Check sheet for the drawn part. Datum: minimum x, y, z corner. Units: mm. A direction names the side the tool comes from. Give positions to 0.01 mm unless a question says otherwise; leave off trailing zeros. Order: outer loops, then holes, each group sorted by start corner. A loop starts at its lowest first (then second) coordinate and runs counter-clockwise, first axis right, second up.
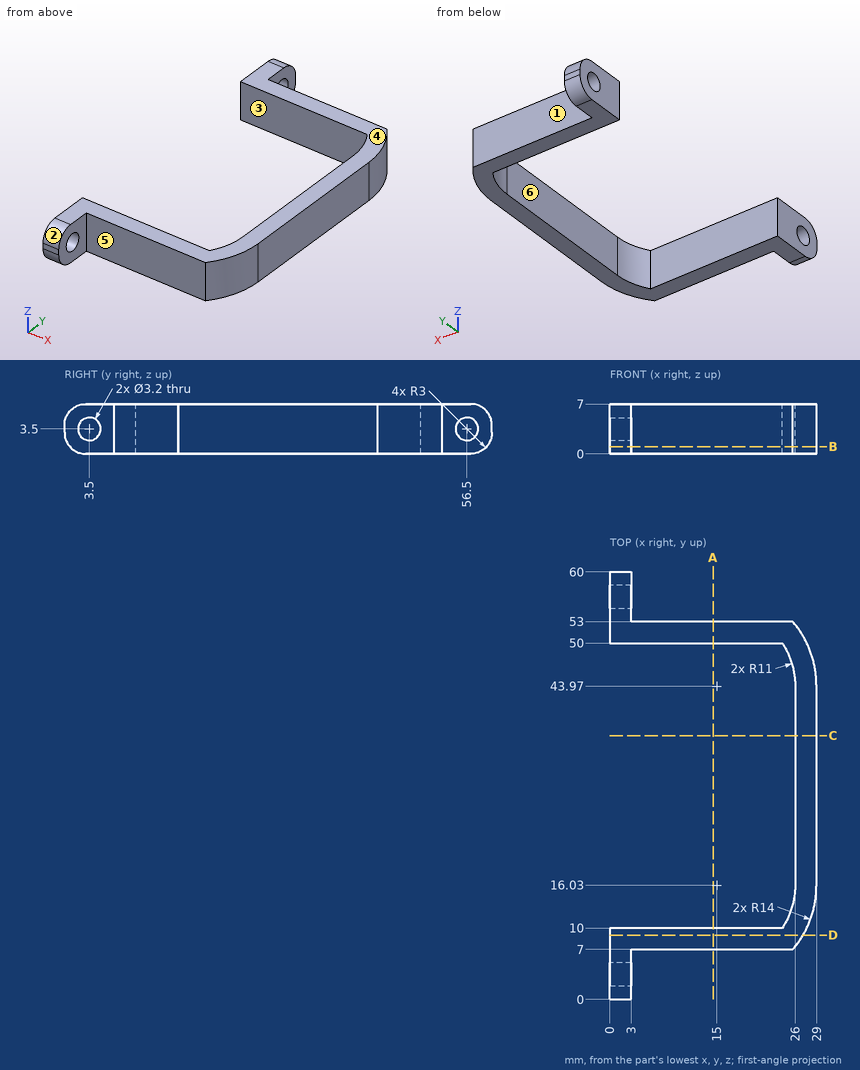
(1) Section check B-B, the plane z = 1. Enter the section's corners in (x, y).
Solved:
outline: (0, 0.76) - (3, 0.76) - (3, 7) - (25.7, 7) arc R14 ccw to (29, 16) - (29, 44) arc R14 ccw to (25.7, 53) - (3, 53) - (3, 59.24) - (0, 59.24) - (0, 50) - (24.2, 50) arc R11 cw to (26, 43.94) - (26, 16.06) arc R11 cw to (24.2, 10) - (0, 10) - close
(2) Section check A-A, the plane x = 14.5. Enter the section's corners in (y, z).
Solved:
outline: (7, 0) - (10, 0) - (10, 7) - (7, 7) - close; (50, 0) - (53, 0) - (53, 7) - (50, 7) - close
(3) Set-up check for the marked faces 4, 5 and 6: record each of +Z, -Z, +X, -X, +Y, -Y from which the full face is reachable in a straight line by a thin tool's end or side.
Solved:
face 4: +Z, +X, -X, +Y, -Y
face 5: +Z, -Z, +X, -Y
face 6: +Z, -Z, -X
(4) Scan lines: line 1 (Y direction, x = 13, z = 6.25); line 2 (Z direction, x = 1.2, y = 56.5); line 3 (X direction, y = 23.5, z = 4.75). Record each from-to range of solid material in increasing order.
Solved:
line 1: y = 7 to 10, 50 to 53
line 2: z = 0 to 1.9, 5.1 to 7
line 3: x = 26 to 29
(5) Go/stop test with flat-tipped pins: pin 1 (2 mm diameter, centred on y = 4, z = 3, fed in from +X); pin 2 (2 mm diameter, centred on x = 13.5, z = 5, fed in from +Y). Record where each tip stops, or that it passes through.
Solved:
pin 1: stops at x = 3
pin 2: stops at y = 53
(6) Section check D-D, the plane y = 9. Enter the section's corners in (x, z), then the cut area to 3 significant figures.
Solved:
outline: (0, 0) - (27.11, 0) - (27.11, 7) - (0, 7) - close
area: 190 mm2
(7) Release check for a two-part mould opening along Y. For the marked faces 1, 2 and 3 record: pulls with the +Y half, pulls with the -Y half, needs draft (parallel to the pull), parting line crosses it, or undercut.
Solved:
face 1: pulls with the +Y half
face 2: pulls with the -Y half
face 3: undercut
(8) Section check C-C, the plane y = 37. Enter the section's corners in (x, z), then the cut area to 3 significant figures.
Solved:
outline: (26, 0) - (29, 0) - (29, 7) - (26, 7) - close
area: 21.0 mm2
